For this review, take the finished solid that the model builds, in its own axes (mm). A direction names the side the tool comes from. Coordinates: 2 decimals unless noted, no trailing zeros. Loops run counter-clockwise (first coordinate to the right, second up) from the corner with the lowest first, then second, coordinate; pieces in that order, holes last. Notation, with made-up numbers: (41.5, 5) - (47.5, 5) arc R25 ccw to (47.5, 28) - close; hole circle Ø10 at (-13.75, 21.25). An arc over 180 degrees is marked (long way). One line per item, written item: value. Start each with the question number.
1. Take a section at A-A, the plane z = -65. State the section outline as (x, y) points, and give its area (3 significant figures).
2. Take a section at B-B, the plane x = 14.5. State the section outline as (y, z) points.
3. Take a section at D-D, the plane x = -9. State the section outline as (y, z) points.
4. To check wall thickness, follow line 1 (X direction, y = 12, z = -7.5); line 2 (X direction, y = 17.25, z = -74); line 3 (X direction, y = 1.5, z = -2). State the ranges of each line that lie inside material, in increasing order. Write a range as from..to.
5. Take a section at C-C, the plane y = 3.5. State the section outline as (x, z) points, and give its area (3 significant figures).
6. For faces 1 (the face through (-23, 10, -42)), 2 (the face through (-10, 15, -69)), 3 (the face through (-10, 10, 14.389)), 4 (the face through (4.59, 10, -41)), list the 3-axis set-ups (+Z, -Z, +X, -X, +Y, -Y) from which the entire face can be reached by the end or side of a thin tool; tool diameter is ignored.
7. Insertion check: pin 1 (6 mm diameter, centred on y = 18, z = -65.5, fed in from +X); pin 2 (6 mm diameter, centred on y = 6.5, z = -67.5, fed in from -X); pin 3 (6 mm diameter, centred on x = -4.5, y = 11, fed in from +Z). Each pin has a flat end and moves straight along its axis. Give the tip position at first contact, or say it passes through.
8. The part is to be moulded in two halves that separate along Y. For faces 5 (the face through (-10, 5, -70)), 6 (the face through (-10, 10, -52)), 7 (the face through (-25.871, 9.86, 3.476)), 8 (the face through (-11, 20, -24)), say which applies: released by +Y, released by -Y, zero draft, split by the parting line, or undercut.
Autodesk Fusion 360 part; units mm, degrees
sketch "Sketch1" plane through (0, 0, 0) normal (0, 1, 0) x (1, 0, 0)
  circle A0 centre (-35.4096, -0.4721) radius 10
  circle A1 centre (14.5882, 0.0008) radius 10
  line L0 (-0.4096, 42) -> (-0.4096, 87)
  line L1 (-20.4096, 87) -> (-20.4096, 42)
  line L2 (-25.429, 39.2855) -> (-25.429, 42)
  line L3 (4.5904, 39.7649) -> (4.5904, 42)
  line L4 (-20.4096, 42) -> (-25.429, 42)
  line L5 (-25.429, 42) -> (-20.4096, 42)
  line L6 (-0.4096, 42) -> (4.5904, 42)
  arc A2 (4.6294, -14.3892) -> (20.7656, 16.3743) centre (14.5882, 0.0008) ccw
  arc A3 (-41.594, 15.8987) -> (-24.8, -14.3892) centre (-35.4096, -0.4721) ccw
  arc A4 (-41.594, 15.8987) -> (-25.429, 39.2855) centre (-50.429, 39.2855) ccw
  arc A5 (4.5904, 39.7649) -> (20.7656, 16.3743) centre (29.5904, 39.7649) ccw
  line L7 (-24.8, -14.3892) -> (4.6294, -14.3892)
  line L8 (-20.4096, 87) -> (-0.4096, 87)
  dimension "d1" = 50
  dimension "d2" = 20
  dimension "d3" = 20
  dimension "d4" = 35
  dimension "d5" = 35
  dimension "d9" = 20
  dimension "d10" = 45
  dimension "d11" = 15
  dimension "d16" = 25
  dimension "d17" = 25
extrude "Extrude1" add sketch "Sketch1" along normal blind 20
sketch "Sketch2" plane through (-0.4096, 0, 0) normal (1, 0, 0) x (0, 1, 0)
  line L0 (0, -42) -> (0, -87)
  line L1 (0, -87) -> (20, -87)
  line L2 (20, -87) -> (20, -42)
  line L3 (20, -42) -> (0, -42)
  line L4 (5, -52) -> (15, -52)
  line L5 (15, -52) -> (15, -87)
  line L6 (15, -87) -> (5, -87)
  line L7 (5, -87) -> (5, -52)
  dimension "d26" = 10
  dimension "d27" = 35
extrude "Extrude2" cut sketch "Sketch2" against normal blind 47.149 contours L1 L4 L5 L6 L7
Solutions:
1. outline: (-20.41, 0) - (-0.41, 0) - (-0.41, 5) - (-20.41, 5) - close; (-20.41, 15) - (-0.41, 15) - (-0.41, 20) - (-20.41, 20) - close
1. area: 200 mm2
2. outline: (0, -19.83) - (20, -19.83) - (20, -10) - (0, -10) - close; (0, 10) - (20, 10) - (20, 17.5) - (0, 17.5) - close
3. outline: (0, -87) - (5, -87) - (5, -52) - (15, -52) - (15, -87) - (20, -87) - (20, 14.39) - (0, 14.39) - close
4. line 1: -50.99..-41.45, -29.37..7.97, 21.2..30.4
4. line 2: -20.41..-0.41
4. line 3: -52.73..-45.1, -25.72..4.79, 24.39..31.97
5. outline: (-41.59, -15.9) arc R25 cw to (-25.43, -39.29) - (-25.43, -42) - (-20.41, -42) - (-20.41, -87) - (-0.41, -87) - (-0.41, -42) - (4.59, -42) - (4.59, -39.76) arc R25 cw to (20.77, -16.37) arc R17.5 ccw (long way) to (4.63, 14.39) - (-24.8, 14.39) arc R17.5 ccw (long way) to start; hole circle Ø20 at (-35.41, 0.47); hole circle Ø20 at (14.59, 0)
5. area: 3,780 mm2
6. face 1: -Z, -X, +Y, -Y
6. face 2: -Z, +X, -X
6. face 3: +Z, +Y, -Y
6. face 4: -Z, +X, +Y, -Y
7. pin 1: x = -0.41
7. pin 2: x = -20.41
7. pin 3: z = 14.39
8. face 5: undercut
8. face 6: undercut
8. face 7: zero draft
8. face 8: released by +Y
